from build123d import *

# Parameters (mm, degrees)
SKETCH1_R           = 37.5
BOSS_EXTRUDE1_DEPTH = 2.61
SKETCH2_R           = 5
CUT_EXTRUDE1_DEPTH  = 13.05
SKETCH3_R           = 1.5
CUT_EXTRUDE2_DEPTH  = 3.61


with BuildPart() as part:
    # Sketch1 → Boss-Extrude1 (new body)
    with BuildSketch(Plane(origin=(0, 0, 0), x_dir=(1, 0, 0), z_dir=(0, 1, 0))):
        Circle(SKETCH1_R)
    extrude(amount=BOSS_EXTRUDE1_DEPTH)

    # Sketch2 → Cut-Extrude1 (cut)
    with BuildSketch(Plane(origin=(0, 2.61, 0), x_dir=(1, 0, 0), z_dir=(0, 1, 0))):
        Circle(SKETCH2_R)
    extrude(amount=-CUT_EXTRUDE1_DEPTH, mode=Mode.SUBTRACT)

    # Sketch3 → Cut-Extrude2 (cut, through all)
    with BuildSketch(Plane(origin=(0, 2.61, 0), x_dir=(1, 0, 0), z_dir=(0, 1, 0))):
        with Locations((-7, 7)):
            Circle(SKETCH3_R)
        with Locations((7, 7)):
            Circle(SKETCH3_R)
        with Locations((7, -7)):
            Circle(SKETCH3_R)
        with Locations((-7, -7)):
            Circle(SKETCH3_R)
    extrude(amount=-CUT_EXTRUDE2_DEPTH, mode=Mode.SUBTRACT)


solid = part.part
Read the model definition and answer for the solid it produces. Units are mm, in the model's axes. Coordinates: 2 decimals unless noted, no trailing zeros. Loops run counter-clockwise (first coordinate to the right, second up) from the corner with the lowest first, then second, coordinate; pieces in that order, holes last.
Q1. The mould has two halves that part along X. Classify faces 1 (the face through (5.8, 1.3, -6.1)), 2 (the face through (8, 0, -1)), 3 (the face through (-4.88, 1.29, -37.18)): +X half, -X half, draft (parallel to the pull), parting line (faces both ways), or undercut.
Q2. Each of these flat-tipped pins is pushed along its axis until it touches: pin 1 Ø2.5 at (x, z) = (7, 7) entering from +Y; pin 2 Ø1.5 at (y, z) = (1, -11) entering from +X; pin 3 Ø1.5 at (y, z) = (0.5, -5.5) entering from +X. Where does it stop, or does it pass through?
Q3. The part is cut by section B-B on y = 2.2. Write down the section's boundary in (x, z), and give its area (3 significant figures).
Q4. The part is cut by section C-C on x = 7. Write down the section's boundary in (y, z), and give its area (3 significant figures).
Q5. The part is cut by section D-D on x = -32. Write down the section's boundary in (y, z).
Q6. The part is cut by section A-A on z = 0. Write down the section's boundary in (x, y).
Q7. Consider probe 1 along Z at (x, y) = (7, 1.2); probe 2 along Z at (x, y) = (0, 1.45). Determine where each line is inside the solid, lowest interval first.
Results below:
1. face 1: undercut
1. face 2: draft
1. face 3: parting line
2. pin 1: passes through
2. pin 2: stops at x = 36.07
2. pin 3: stops at x = 37.2
3. outline: circle Ø75 at (0, 0); hole circle Ø3 at (-7, -7); hole circle Ø3 at (-7, 7); hole circle Ø10 at (0, 0); hole circle Ø3 at (7, -7); hole circle Ø3 at (7, 7)
3. area: 4,310 mm2
4. outline: (0, -36.84) - (2.61, -36.84) - (2.61, -8.5) - (0, -8.5) - close; (0, -5.5) - (2.61, -5.5) - (2.61, 5.5) - (0, 5.5) - close; (0, 8.5) - (2.61, 8.5) - (2.61, 36.84) - (0, 36.84) - close
4. area: 177 mm2
5. outline: (0, -19.55) - (2.61, -19.55) - (2.61, 19.55) - (0, 19.55) - close
6. outline: (-37.5, 0) - (-5, 0) - (-5, 2.61) - (-37.5, 2.61) - close; (5, 0) - (37.5, 0) - (37.5, 2.61) - (5, 2.61) - close
7. probe 1: z = -36.84 to -8.5, -5.5 to 5.5, 8.5 to 36.84
7. probe 2: z = -37.5 to -5, 5 to 37.5
